Here's how the part is built. I have some questions about the finished solid (model axes, mm). A direction names the side the tool comes from. Round coordinates to 2 decimals unless told otherwise and drop trailing zeros. Write each loop counter-clockwise with the first axis right and the second up, starting at its lowest first coordinate (ties: lowest second). Pieces come first, ordered by that corner, then holes. Notation, with made-up numbers: (77.25, 1) -> (133.25, 1) arc R23 ccw to (133.25, 10) -> close; hole circle Ø1 at (-14, 54). An arc over 180 degrees is marked (long way). Put each result on its own line as item: value. Start each with the question number.
1. Suppose I cut it at A-A (y = 0). Please give me the cut outline in (x, z).
2. I need wall thicknesses on probe 1 along Y at (x, z) = (0, -4.5); probe 2 along X at (y, z) = (-41.65, -1.35); probe 3 along Y at (x, z) = (1, 5.5). Which ranges of each line are inside material? Lowest first, please. Write a range as from..to.
3. Suppose I cut it at C-C (z = -1.5). Count the separate pieces of the cut face and the enclosed holes in it, then the cut area to 3 significant figures.
4. For pin 1 (4 mm diameter, centred on x = 15.5, y = -41.65, fed in from +Z); pin 2 (3 mm diameter, centred on x = 14, y = -71.5, fed in from -Z); pin 3 (10 mm diameter, centred on x = -28.575, y = -85.725, fed in from +Z) (3 decimals); pin 4 (4 mm diameter, centred on x = -27, z = 1, fed in from +Y), each with a flat end and sliding along its axis, tell me the tip position at first contact or that it passes through.
5. We'd pull the mould along Y, two halves only. Please class faces 4 (the face through (-1, -95.25, 0)), 5 (the face through (0, 38.1, 0)), 6 (the face through (-21.191, -57, 3)): +Y half, -Y half, draft (parallel to the pull), parting line (faces both ways), or undercut.
6. Suppose I cut it at B-B (x = 27.5). Please give me the cut outline in (y, z) (3 decimals).
7. Which directions (+Z, -Z, +X, -X, +Y, -Y) give clear straight access to the entire face, cutting with the end or side of a thin tool? Please do faces 1 (the face through (15.721, -70.964, -1.698)), 2 (the face through (14, -43, -3.35)), 3 (the face through (32.2, -85.6, 1.905)).
8. Suppose I cut it at D-D (y = -57.15). Please give me the cut outline in (x, z), then the cut area to 3 significant figures.
```python
from build123d import *

# Parameters (mm, degrees)
SKETCH2_W                                        = 76.2
SKETCH2_H                                        = 133.35
BOSS_EXTRUDE1_DEPTH                              = 6.35
F_3_8_CLEARANCE_HOLE1_D                          = 10.0838
M3_CLEARANCE_HOLE1_D                             = 3.4
SKETCH13_R                                       = 12.7
CUT_EXTRUDE2_DEPTH                               = 13.7
SKETCH14_W                                       = 42.381000074
SKETCH14_H                                       = 42.381000074
CUT_EXTRUDE3_DEPTH                               = 6.35
CHAMFER1_SIZE                                    = 25.4
CBORE_FOR_1_4_SOCKET_HEAD_CAP_SCREW1_D           = 6.7564
CBORE_FOR_1_4_SOCKET_HEAD_CAP_SCREW1_CBORE_D     = 11.1125
CBORE_FOR_1_4_SOCKET_HEAD_CAP_SCREW1_CBORE_DEPTH = 4.445
CBORE_FOR_M3_SHCS1_D                             = 3.4
CBORE_FOR_M3_SHCS1_CBORE_D                       = 6.5
CBORE_FOR_M3_SHCS1_CBORE_DEPTH                   = 3
FILLET1_R                                        = 6.35
FILLET2_R                                        = 12.7


with BuildPart() as part:
    # Sketch2 → Boss-Extrude1 (new body, symmetric)
    with BuildSketch(Plane.XY):
        with Locations((0, -28.575)):
            Rectangle(SKETCH2_W, SKETCH2_H)
    extrude(amount=BOSS_EXTRUDE1_DEPTH, both=True)

    # 3/8 Clearance Hole1 (through all)
    with Locations(Plane.XY.offset(6.35)):
        with Locations((0, 0)):
            Hole(F_3_8_CLEARANCE_HOLE1_D / 2)

    # M3 Clearance Hole1 (through all)
    with Locations(Plane.XY.offset(6.35)):
        with Locations((-15.5, -41.65), (15.5, -41.65), (15.5, -72.65), (-15.5, -72.65)):
            Hole(M3_CLEARANCE_HOLE1_D / 2)

    # Sketch13 → Cut-Extrude2 (cut, through all)
    with BuildSketch(Plane.XY.offset(6.35)):
        with Locations((0, -57.15)):
            Circle(SKETCH13_R)
    extrude(amount=-CUT_EXTRUDE2_DEPTH, mode=Mode.SUBTRACT)

    # Sketch14 → Cut-Extrude3 (cut)
    with BuildSketch(Plane.XY.offset(6.35)):
        with Locations((0, -57.15)):
            Rectangle(SKETCH14_W, SKETCH14_H)
    extrude(amount=-CUT_EXTRUDE3_DEPTH, mode=Mode.SUBTRACT)

    # Chamfer1
    chamfer1_edges = [part.edges().sort_by_distance(p)[0] for p in [
        (-38.1, 38.1, 0),
        (38.1, 38.1, 0),
    ]]
    chamfer(chamfer1_edges, length=CHAMFER1_SIZE)

    # CBORE for 1/4 Socket Head Cap Screw1 (through all)
    with Locations(Plane.XY.offset(6.35)):
        with Locations((-28.575, -85.725), (28.575, -85.725)):
            CounterBoreHole(CBORE_FOR_1_4_SOCKET_HEAD_CAP_SCREW1_D / 2, CBORE_FOR_1_4_SOCKET_HEAD_CAP_SCREW1_CBORE_D / 2, CBORE_FOR_1_4_SOCKET_HEAD_CAP_SCREW1_CBORE_DEPTH)

    # CBORE for M3 SHCS1 (through all)
    with Locations(Plane(origin=(0, 0, -6.35), x_dir=(-1, 0, 0), z_dir=(0, 0, -1))):
        with Locations((-15.5, -41.65), (15.5, -41.65), (15.5, -72.65), (-15.5, -72.65)):
            CounterBoreHole(CBORE_FOR_M3_SHCS1_D / 2, CBORE_FOR_M3_SHCS1_CBORE_D / 2, CBORE_FOR_M3_SHCS1_CBORE_DEPTH)

    # Fillet1
    fillet1_edges = [part.edges().sort_by_distance(p)[0] for p in [
        (-21.190500037, -35.959499963, 3.175),
        (-21.190500037, -78.340500037, 3.175),
        (21.190500037, -78.340500037, 3.175),
        (21.190500037, -35.959499963, 3.175),
    ]]
    fillet(fillet1_edges, radius=FILLET1_R)

    # Fillet2
    fillet2_edges = [part.edges().sort_by_distance(p)[0] for p in [
        (-12.7, 38.1, 0),
        (12.7, 38.1, 0),
        (38.1, 12.7, 0),
        (-38.1, 12.7, 0),
    ]]
    fillet(fillet2_edges, radius=FILLET2_R)


solid = part.part
```
Verdict:
1. outline: (-38.1, -6.35) -> (-5.04, -6.35) -> (-5.04, 6.35) -> (-38.1, 6.35) -> close; (5.04, -6.35) -> (38.1, -6.35) -> (38.1, 6.35) -> (5.04, 6.35) -> close
2. probe 1: y = -95.25..-69.85, -44.45..-5.04, 5.04..38.1
2. probe 2: x = -38.1..-17.2, -13.8..13.8, 17.2..38.1
2. probe 3: y = -95.25..-78.34, -35.96..-4.94, 4.94..38.1
3. separate pieces: 1
3. enclosed holes: 8
3. area: 8,810 mm^2
4. pin 1: stops at z = 0
4. pin 2: stops at z = -6.35
4. pin 3: stops at z = 1.905
4. pin 4: stops at y = 25.8
5. face 4: -Y half
5. face 5: +Y half
5. face 6: undercut
6. outline: (-95.25, -6.35) -> (-88.928, -6.35) -> (-88.928, 1.905) -> (-91.176, 1.905) -> (-91.176, 6.35) -> (-95.25, 6.35) -> close; (-82.522, -6.35) -> (23.3, -6.35) -> (23.3, 6.35) -> (-80.274, 6.35) -> (-80.274, 1.905) -> (-82.522, 1.905) -> close
7. face 1: +Z, -Z
7. face 2: -Z
7. face 3: +Z
8. outline: (-38.1, -6.35) -> (-12.7, -6.35) -> (-12.7, 0) -> (-21.19, 0) -> (-21.19, 6.35) -> (-38.1, 6.35) -> close; (12.7, -6.35) -> (38.1, -6.35) -> (38.1, 6.35) -> (21.19, 6.35) -> (21.19, 0) -> (12.7, 0) -> close
8. area: 537 mm^2
